from build123d import *

# Parameters (mm, degrees)
SKETCH1_W               = 80
SKETCH1_H               = 80
SKETCH1_R               = 18.4
BOSS_EXTRUDE1_DEPTH     = 2
SKETCH2_W               = 4
SKETCH2_H               = 18.5
BOSS_EXTRUDE2_DEPTH     = 15.25
SKETCH3_R               = 2.2
CUT_EXTRUDE1_DEPTH      = 94.976393312
MIRROR2_COPY_1_SKETCH_W = 4
MIRROR2_COPY_1_SKETCH_H = 18.5
MIRROR2_COPY_1_DEPTH    = 15.25
MIRROR2_COPY_2_SKETCH_R = 2.2
MIRROR2_COPY_2_DEPTH    = 94.976393312
SKETCH4_R               = 2.2
CUT_EXTRUDE2_DEPTH      = 62.388618652
SKETCH5_W               = 4
SKETCH5_H               = 15.25
CUT_EXTRUDE3_DEPTH      = 93.258129723
SKETCH6_W               = 80
SKETCH6_H               = 80
SKETCH6_W_2             = 76
SKETCH6_H_2             = 76
BOSS_EXTRUDE3_DEPTH     = 75
SKETCH7_W               = 25
SKETCH7_H               = 77
BOSS_EXTRUDE4_DEPTH     = 80
CUT_EXTRUDE5_DEPTH      = 21


with BuildPart() as part:
    # Sketch1 → Boss-Extrude1 (new body)
    with BuildSketch(Plane(origin=(0, 0, 0), x_dir=(1, 0, 0), z_dir=(0, 1, 0))):
        Rectangle(SKETCH1_W, SKETCH1_H)
        with Locations(Location((0, 0, 0), (0, 0, 270))):
            Circle(SKETCH1_R, mode=Mode.SUBTRACT)
    extrude(amount=BOSS_EXTRUDE1_DEPTH)

    # Sketch2 → Boss-Extrude2 (add)
    with BuildSketch(Plane(origin=(0, 2, 0), x_dir=(1, 0, 0), z_dir=(0, 1, 0))):
        with Locations((42, -30.75)):
            Rectangle(SKETCH2_W, SKETCH2_H)
    boss_extrude2 = extrude(amount=-BOSS_EXTRUDE2_DEPTH)

    # Sketch3 → Cut-Extrude1 (cut, through all)
    with BuildSketch(Plane(origin=(44, 0, 0), x_dir=(0, 0, -1), z_dir=(1, 0, 0))):
        with Locations((-30.75, -8.125)):
            Circle(SKETCH3_R)
    cut_extrude1 = extrude(amount=-CUT_EXTRUDE1_DEPTH, mode=Mode.SUBTRACT)

    # Mirror1: Boss-Extrude2, Cut-Extrude1 across plane
    add(boss_extrude2.mirror(Plane(origin=(0, 0, 0), x_dir=(0, 0, 1), z_dir=(1, 0, 0))))
    add(cut_extrude1.mirror(Plane(origin=(0, 0, 0), x_dir=(0, 0, 1), z_dir=(1, 0, 0))), mode=Mode.SUBTRACT)

    # Mirror2: Boss-Extrude2, Cut-Extrude1 across plane
    add(boss_extrude2.mirror(Plane(origin=(0, 0, 0), x_dir=(1, 0, 0), z_dir=(0, 0, -1))))
    add(cut_extrude1.mirror(Plane(origin=(0, 0, 0), x_dir=(1, 0, 0), z_dir=(0, 0, -1))), mode=Mode.SUBTRACT)

    # Mirror2 copy 1 sketch → Mirror2 copy 1 (add)
    with BuildSketch(Plane(origin=(0, 2, 0), x_dir=(-1, 0, 0), z_dir=(0, 1, 0))):
        with Locations((42, -30.75)):
            Rectangle(MIRROR2_COPY_1_SKETCH_W, MIRROR2_COPY_1_SKETCH_H)
    extrude(amount=-MIRROR2_COPY_1_DEPTH)

    # Mirror2 copy 2 sketch → Mirror2 copy 2 (cut, through all)
    with BuildSketch(Plane.ZY.offset(44)):
        with Locations((-30.75, -8.125)):
            Circle(MIRROR2_COPY_2_SKETCH_R)
    extrude(amount=-MIRROR2_COPY_2_DEPTH, mode=Mode.SUBTRACT)

    # Sketch4 → Cut-Extrude2 (cut, through all)
    with BuildSketch(Plane(origin=(0, 2, 0), x_dir=(1, 0, 0), z_dir=(0, 1, 0))):
        with Locations(Location((-24, 24, 0), (0, 0, 270))):
            Circle(SKETCH4_R)
        with Locations(Location((24, 24, 0), (0, 0, 270))):
            Circle(SKETCH4_R)
    cut_extrude2 = extrude(amount=-CUT_EXTRUDE2_DEPTH, mode=Mode.SUBTRACT)

    # Mirror3: Cut-Extrude2 across plane
    add(cut_extrude2.mirror(Plane(origin=(0, 0, 0), x_dir=(1, 0, 0), z_dir=(0, 0, -1))), mode=Mode.SUBTRACT)

    # Sketch5 → Cut-Extrude3 (cut, through all)
    with BuildSketch(Plane.XY.offset(40)):
        with Locations((-42, -5.625)):
            Rectangle(SKETCH5_W, SKETCH5_H)
        with Locations((42, -5.625)):
            Rectangle(SKETCH5_W, SKETCH5_H)
    extrude(amount=-CUT_EXTRUDE3_DEPTH, mode=Mode.SUBTRACT)

    # Sketch6 → Boss-Extrude3 (add)
    with BuildSketch(Plane(origin=(0, 2, 0), x_dir=(1, 0, 0), z_dir=(0, 1, 0))):
        Rectangle(SKETCH6_W, SKETCH6_H)
        Rectangle(SKETCH6_W_2, SKETCH6_H_2, mode=Mode.SUBTRACT)
    extrude(amount=BOSS_EXTRUDE3_DEPTH)

    # Sketch7 → Boss-Extrude4 (add)
    with BuildSketch(Plane.XY.offset(40)):
        with Locations((-52.5, 38.5)):
            Rectangle(SKETCH7_W, SKETCH7_H)
        with Locations((52.5, 38.5)):
            Rectangle(SKETCH7_W, SKETCH7_H)
    extrude(amount=-BOSS_EXTRUDE4_DEPTH)

    # Sketch9 → Cut-Extrude5 (cut)
    with BuildSketch(Plane(origin=(65, 0, 0), x_dir=(0, 0, -1), z_dir=(1, 0, 0))):
        Polygon((40, 0), (40, 28), (12, 0), align=None)
    cut_extrude5 = extrude(amount=-CUT_EXTRUDE5_DEPTH, mode=Mode.SUBTRACT)

    # Mirror4: Cut-Extrude5 across plane
    add(cut_extrude5.mirror(Plane(origin=(0, 0, 0), x_dir=(0, 0, 1), z_dir=(1, 0, 0))), mode=Mode.SUBTRACT)


solid = part.part
Geometry: final body of the model. Coordinates: model frame, mm. A direction names the side the tool comes from. Round coordinates to 2 decimals unless told otherwise and drop trailing zeros. Write each loop counter-clockwise with the first axis right and the second up, starting at its lowest first coordinate (ties: lowest second). Pieces come first, ordered by that corner, then holes. Notation, with made-up numbers: M -38.75,-37.75 L -19.75,-37.75 A18 cw -19.75,-12.75 Z; hole C 85.5,26.25 d6. An arc over 180 degrees is marked long. Write item = value, one per line.
Item 1: Access query for faces 4 (the face through (-44, 77, 1)), 5 (the face through (38, 39, 1)), 6 (the face through (44, 8, -32)). Directions: +Z, -Z, +X, -X, +Y, -Y. A direction counts if a zero-diameter tool reaches every point of the face in a straight line with its end or side. Return the directions, or none.
Findings:
face_4 = +Z, -Z, +X, -X, +Y
face_5 = +Y
face_6 = -Z, +X, -Y
Item 2: Section query A-A on z = -24. Return loops of the section in (x, y), then the cut area to 3 significant figures.
Findings:
outline = M -65,12 L -44,12 L -44,0 L -26.2,0 L -26.2,2 L -38,2 L -38,77 L -65,77 Z; M -21.8,0 L 21.8,0 L 21.8,2 L -21.8,2 Z; M 26.2,0 L 44,0 L 44,12 L 65,12 L 65,77 L 38,77 L 38,2 L 26.2,2 Z
area = 3,790 mm^2
Item 3: Pin query (flat end, axial travel): P1, Ø5, axis at y = 8.5, z = -26.5, coming from the -X side; P2, Ø8, axis at x = -30, z = -9.5, coming from the +Y side. Return the tip coordinate at first contact, or that it passes through.
Findings:
P1 = -44
P2 = 2
Item 4: Pull-direction query (X, two-part tool) for faces 1 (the face through (-44, 8, -32)), 2 (the face through (-1, 39, -38)), 3 (the face through (-55, 14, -26)); classes: pulls with the +X half, pulls with the -X half, needs draft (parallel to the pull), parting line crosses it, or undercut.
Findings:
face_1 = pulls with the -X half
face_2 = undercut
face_3 = needs draft
Item 5: Section query C-C on y = 38. Return loops of the section in (x, z).
Findings:
outline = M -65,-40 L 65,-40 L 65,40 L -65,40 Z; hole M -38,-38 L 38,-38 L 38,38 L -38,38 Z
Item 6: Section query B-B on x = 0. Return loops of the section in (y, z), then the cut area to 3 significant figures.
Findings:
outline = M 0,-40 L 77,-40 L 77,-38 L 2,-38 L 2,-18.4 L 0,-18.4 Z; M 0,18.4 L 2,18.4 L 2,38 L 77,38 L 77,40 L 0,40 Z
area = 386 mm^2
Item 7: Material intervals for line 1 along X through (y, z) = (1, -24); line 2 along X through (y, z) = (67, 21); line 3 along X through (y, z) = (0.85, 0), sorted ascending. Write a range as [from, to].
Findings:
line_1 = [-44, -26.2], [-21.8, 21.8], [26.2, 44]
line_2 = [-65, -38], [38, 65]
line_3 = [-65, -18.4], [18.4, 65]
Item 8: Section query D-D on x = 24. Return loops of the section in (y, z), then the cut area to 3 significant figures.
Findings:
outline = M 0,-40 L 77,-40 L 77,-38 L 2,-38 L 2,-26.2 L 0,-26.2 Z; M 0,-21.8 L 2,-21.8 L 2,21.8 L 0,21.8 Z; M 0,26.2 L 2,26.2 L 2,38 L 77,38 L 77,40 L 0,40 Z
area = 442 mm^2
